Input: part model. Units: mm. Frame: model coordinates. Coordinates: 2 decimals unless noted, no trailing zeros. Loops run counter-clockwise (first coordinate to the right, second up) from the corner with the lowest first, then second, coordinate; pieces in that order, holes last.
Item 1: Section B-B on z = -11. Return loops of the section in (x, y), and give its area (3 significant figures).
Item 2: Section C-C on x = -32. Return loops of the section in (y, z).
Item 3: Ray query, line 1 along X through (y, z) = (-12, 50.8); line 2 along X through (y, z) = (-16.25, 1.5); line 3 along Z through (x, y) = (-25, -22.5). Return the intervals inside material, ascending.
Item 4: Pull-direction query (X, two-part tool) for faces 1 (the cylindrical face through (-44.541, -12.522, 60.323)), 2 (the flat face through (-42, 0, -20)), 3 (the flat face through (-28.858, -13, -24)), 4 (the cylindrical face through (-47.46, -12.52, 36.01)); classes: released by +X, released by -X, zero draft, split by the parting line, or undercut.
Item 5: Contact query for flat-ended pins moving along their axis: P1, Ø3, axis at x = -48.97, z = 35.53, coming from the +Y side; P2, Ø10, axis at x = -32, y = -2.5, coming from the +Z side; P3, Ø5, axis at y = -15, z = 14, coming from the -X side; P4, Ø10, axis at y = -16, z = -30, coming from the +X side. Output: stop coordinate, or through.
```python
from build123d import *

# Parameters (mm, degrees)
F0_R     = 1.5875
F1_DEPTH = 25.4


with BuildPart() as f1:
    # F0 (on Front) → F1 (new body)
    with BuildSketch(Plane.XZ):
        with BuildLine():
            ThreePointArc((-44.7390819472, 41.2750016461), (-44.7348827118, 41.341553676), (-44.7334821429, 41.4082233443))
            Line((-44.7334821429, 41.4082233443), (-44.7334821429, 41.275))
            ThreePointArc((-44.7334821429, 41.275), (-37.9982900521, 44.0648079092), (-35.2084821429, 50.8))
            ThreePointArc((-35.2084821429, 50.8), (-35.2271772486, 51.396483242), (-35.2831891786, 51.990625))
            ThreePointArc((-35.2831891786, 51.990625), (-44.7334821429, 60.325), (-54.1837751071, 51.990625))
            ThreePointArc((-54.1837751071, 51.990625), (-51.8790837955, 44.5019048894), (-44.7390819472, 41.2750016461))
        make_face()
        with BuildLine():
            ThreePointArc((-41.5584821429, 50.8), (-42.4884181126, 48.5549359697), (-44.7334821429, 47.625))
            ThreePointArc((-44.7334821429, 47.625), (-46.9785461731, 53.0450640303), (-41.5584821429, 50.8))
        make_face(mode=Mode.SUBTRACT)
        with BuildLine():
            ThreePointArc((-35.2084821429, 50.8), (-37.9982900521, 44.0648079092), (-44.7334821429, 41.275))
            Line((-44.7334821429, 41.275), (-44.7334821429, 15.875))
            ThreePointArc((-44.7334821429, 15.875), (-34.2331566271, 11.90625), (-28.9829938692, 1.984375))
            Line((-28.9829938692, 1.984375), (-35.2831891786, 51.990625))
            ThreePointArc((-35.2831891786, 51.990625), (-35.2271772486, 51.396483242), (-35.2084821429, 50.8))
        make_face()
        with BuildLine():
            Line((-44.7334821429, 15.875), (-44.7334821429, 41.275))
            ThreePointArc((-44.7334821429, 41.275), (-44.7362820451, 41.2750004115), (-44.7390819472, 41.2750016461))
            ThreePointArc((-44.7390819472, 41.2750016461), (-51.8790837955, 44.5019048894), (-54.1837751071, 51.990625))
            Line((-54.1837751071, 51.990625), (-60.4839704165, 1.984375))
            ThreePointArc((-60.4839704165, 1.984375), (-55.2338076586, 11.90625), (-44.7334821429, 15.875))
        make_face()
        with Locations((-48.9732250571, 35.5329811573)):
            Circle(F0_R, mode=Mode.SUBTRACT)
        with BuildLine():
            ThreePointArc((-28.9829938692, 1.984375), (-34.2331566271, 11.90625), (-44.7334821429, 15.875))
            Line((-44.7334821429, 15.875), (-44.7334821429, 3.175))
            ThreePointArc((-44.7334821429, 3.175), (-42.4884181126, 2.2450640303), (-41.5584821429, 0))
            ThreePointArc((-41.5584821429, 0), (-42.4884181126, -2.2450640303), (-44.7334821429, -3.175))
            Line((-44.7334821429, -3.175), (-44.7334821429, -15.875))
            ThreePointArc((-44.7334821429, -15.875), (-33.5081619915, -11.2253201513), (-28.8584821429, 0))
            ThreePointArc((-28.8584821429, 0), (-28.8896406525, 0.9941387366), (-28.9829938692, 1.984375))
        make_face()
        with BuildLine():
            Line((-44.7334821429, 3.175), (-44.7334821429, 15.875))
            ThreePointArc((-44.7334821429, 15.875), (-55.2338076586, 11.90625), (-60.4839704165, 1.984375))
            ThreePointArc((-60.4839704165, 1.984375), (-60.6072259583, 0.1997054867), (-60.5289077069, -1.5875))
            ThreePointArc((-60.5289077069, -1.5875), (-55.3827558857, -11.7732150983), (-44.7334821429, -15.875))
            Line((-44.7334821429, -15.875), (-44.7334821429, -3.175))
            ThreePointArc((-44.7334821429, -3.175), (-47.9084821429, 0), (-44.7334821429, 3.175))
        make_face()
        with BuildLine():
            Line((-28.8584821429, -46.8677527116), (-28.8584821429, 0))
            ThreePointArc((-28.8584821429, 0), (-33.5081619915, -11.2253201513), (-44.7334821429, -15.875))
            Line((-44.7334821429, -15.875), (-44.7334821429, -53.975))
            ThreePointArc((-44.7334821429, -53.975), (-44.7300940156, -53.9750006026), (-44.7267058887, -53.9750024104))
            ThreePointArc((-44.7267058887, -53.9750024104), (-44.3934690624, -53.9810706429), (-44.060648545, -53.9987937634))
            ThreePointArc((-44.060648545, -53.9987937634), (-37.7644662504, -57.0070467051), (-35.2084821429, -63.5))
            Line((-35.2084821429, -63.5), (-8.2209821429, -63.5))
            ThreePointArc((-8.2209821429, -63.5), (-5.8961422185, -57.8873399243), (-0.2834821429, -55.5625))
            Line((-0.2834821429, -55.5625), (-21.1931293796, -54.8128481856))
            ThreePointArc((-21.1931293796, -54.8128481856), (-26.6297449166, -52.3877657341), (-28.8584821429, -46.8677527116))
        make_face()
        with BuildLine():
            ThreePointArc((-44.7334821429, -15.875), (-55.3827558857, -11.7732150983), (-60.5289077069, -1.5875))
            Line((-60.5289077069, -1.5875), (-54.2107374813, -64.4525))
            ThreePointArc((-54.2107374813, -64.4525), (-51.7974112018, -57.1104357543), (-44.7334821429, -53.975))
            Line((-44.7334821429, -53.975), (-44.7334821429, -15.875))
        make_face()
        with BuildLine():
            ThreePointArc((-44.7334821429, -53.975), (-51.7974112018, -57.1104357543), (-54.2107374813, -64.4525))
            ThreePointArc((-54.2107374813, -64.4525), (-50.9958655245, -70.6769199091), (-44.3933035714, -73.0189234444))
            ThreePointArc((-44.3933035714, -73.0189234444), (-37.8790738572, -70.1138273378), (-35.2084821429, -63.5))
            Line((-35.2084821429, -63.5), (-41.5584821429, -63.5))
            ThreePointArc((-41.5584821429, -63.5), (-46.9785461731, -65.7450640303), (-44.7334821429, -60.325))
            Line((-44.7334821429, -60.325), (-44.7334821429, -53.975))
        make_face()
        with BuildLine():
            ThreePointArc((-35.2084821429, -63.5), (-37.8790738572, -70.1138273378), (-44.3933035714, -73.0189234444))
            Line((-44.3933035714, -73.0189234444), (0, -71.4324362036))
            ThreePointArc((0, -71.4324362036), (-5.7950049243, -69.2120069047), (-8.2209821429, -63.5))
            Line((-8.2209821429, -63.5), (-35.2084821429, -63.5))
        make_face()
        with BuildLine():
            ThreePointArc((7.6540178571, -63.5), (5.3291779328, -57.8873399243), (-0.2834821429, -55.5625))
            ThreePointArc((-0.2834821429, -55.5625), (-5.8961422185, -57.8873399243), (-8.2209821429, -63.5))
            ThreePointArc((-8.2209821429, -63.5), (-5.7950049243, -69.2120069047), (0, -71.4324362036))
            ThreePointArc((0, -71.4324362036), (5.4285247619, -69.0115227815), (7.6540178571, -63.5))
        make_face()
        with BuildLine():
            ThreePointArc((-44.7267058887, -53.9750024104), (-44.7300940156, -53.9750006026), (-44.7334821429, -53.975))
            Line((-44.7334821429, -53.975), (-44.7334821429, -60.325))
            ThreePointArc((-44.7334821429, -60.325), (-42.4884181126, -61.2549359697), (-41.5584821429, -63.5))
            Line((-41.5584821429, -63.5), (-35.2084821429, -63.5))
            ThreePointArc((-35.2084821429, -63.5), (-37.7644662504, -57.0070467051), (-44.060648545, -53.9987937634))
            Line((-44.060648545, -53.9987937634), (-44.7267058887, -53.9750024104))
        make_face()
    extrude(amount=F1_DEPTH)


solid = f1.part
```
Results found:
1. outline: (-59.58, -25.4) - (-28.86, -25.4) - (-28.86, 0) - (-59.58, 0) - close
1. area: 780 mm2
2. outline: (-25.4, -72.58) - (0, -72.58) - (0, 25.93) - (-25.4, 25.93) - close
3. line 1: x = -54.33 to -47.91, -41.56 to -35.13
3. line 2: x = -60.54 to -47.53, -41.94 to -28.93
3. line 3: z = -72.33 to -53.68
4. face 1: split by the parting line
4. face 2: zero draft
4. face 3: released by +X
4. face 4: undercut
5. P1: passes through
5. P2: stops at z = 56.36
5. P3: stops at x = -59.29
5. P4: stops at x = -28.86
